Geometry check sheet. Reference: the model listing, model coordinates, mm. Coordinates: 2 decimals unless noted, no trailing zeros. Write each loop counter-clockwise with the first axis right and the second up, starting at its lowest first coordinate (ties: lowest second). Pieces come first, ordered by that corner, then holes. Notation, with made-up numbers: M 32,64.5 L 51,64.5 A25 cw 51,92.5 Z; hole C 41,-29 d3. An arc over 180 degrees is marked long. Write each question's results on one line, items separated by ' | '.
```python
from build123d import *

# Parameters (mm, degrees)
SKETCH_1_W      = 55
SKETCH_1_H      = 90
SKETCH_1_R      = 1.5
EXTRUDE_1_DEPTH = 3
FILLET_1_R      = 1


with BuildPart() as part:
    # 草图1 → 凸台-拉伸1 (new body)
    with BuildSketch(Plane(origin=(0, 0, 0), x_dir=(1, 0, 0), z_dir=(0, 1, 0))):
        with Locations((27.5, -45)):
            Rectangle(SKETCH_1_W, SKETCH_1_H)
        with Locations(Location((17.5, -11, 0), (0, 0, 270))):
            Circle(SKETCH_1_R, mode=Mode.SUBTRACT)
        with Locations(Location((51, -10, 0), (0, 0, 270))):
            Circle(SKETCH_1_R, mode=Mode.SUBTRACT)
        with Locations(Location((21, -70, 0), (0, 0, 270))):
            Circle(SKETCH_1_R, mode=Mode.SUBTRACT)
        with Locations(Location((51, -70, 0), (0, 0, 270))):
            Circle(SKETCH_1_R, mode=Mode.SUBTRACT)
    extrude(amount=EXTRUDE_1_DEPTH)

    # 圆角1
    fillet_1_edges = [part.edges().sort_by_distance(p)[0] for p in [
        (0, 1.5, 0),
        (55, 1.5, 0),
        (55, 1.5, 90),
        (0, 1.5, 90),
    ]]
    fillet(fillet_1_edges, radius=FILLET_1_R)


solid = part.part
```
Q1. Sectioned sample at C-C on z = 70. Record the cut outline in (x, y), and give its area (3 significant figures).
Geometry check:
outline: M 0,0 L 19.5,0 L 19.5,3 L 0,3 Z; M 22.5,0 L 49.5,0 L 49.5,3 L 22.5,3 Z; M 52.5,0 L 55,0 L 55,3 L 52.5,3 Z | area: 147 mm2
Q2. Sectioned sample at A-A on x = 17.5. Record the cut outline in (y, z).
Geometry check:
outline: M 0,0 L 3,0 L 3,9.5 L 0,9.5 Z; M 0,12.5 L 3,12.5 L 3,90 L 0,90 Z
Q3. Sectioned sample at B-B on x = 51. Record the cut outline in (y, z), and give its area (3 significant figures).
Geometry check:
outline: M 0,0 L 3,0 L 3,8.5 L 0,8.5 Z; M 0,11.5 L 3,11.5 L 3,68.5 L 0,68.5 Z; M 0,71.5 L 3,71.5 L 3,90 L 0,90 Z | area: 252 mm2
Q4. Mould release check, pull along Z, two halves, no side actions. Record for faces 1 (the flat face through (27, 1, 0)), 2 (the cylindrical face through (49.536, 1.479, 9.675)), 3 (the cylindrical face through (21.45, 1.48, 71.43)), 4 (the flat face through (0, 1, 46)): pulls with the +Z half, pulls with the -Z half, needs draft (parallel to the pull), parting line crosses it, or undercut.
Geometry check:
face 1: pulls with the -Z half | face 2: undercut | face 3: undercut | face 4: needs draft
Q5. Scan lines: probe 1 along X at (y, z) = (2, 70); probe 2 along X at (y, z) = (1.4, 11). Record each from-to range of solid material in increasing order.
Geometry check:
probe 1: x = 0 to 19.5, 22.5 to 49.5, 52.5 to 55 | probe 2: x = 0 to 16, 19 to 49.88, 52.12 to 55
